For this review, use the dimensioned drawing (mm, ordinates from the lowest corner) and the shaded views. Give positions to 0.01 mm unless a question says otherwise; leave off trailing zeros. Order: outer loops, then holes, each group sorted by start corner. A loop starts at its lowest first (then second) coordinate and runs counter-clockwise, first axis right, second up. Notation, with made-up numbers: (-11.5, 26.5) - (9.5, 26.5) arc R15 cw to (9.5, 55.5) - close; hole circle Ø11 at (33, 66). An arc over 180 degrees is marked (long way). Answer as CSV lines item,"result". Start each with the question number.
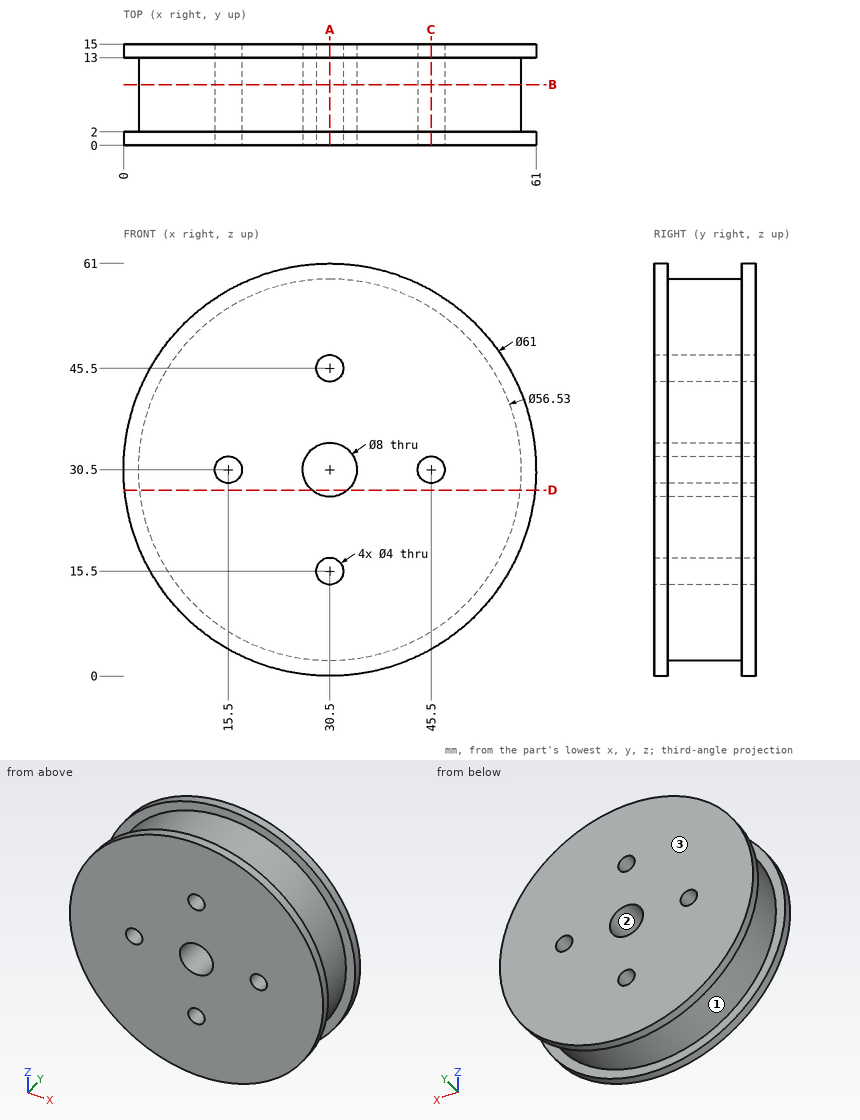
Item 1: For line 1 along X through (y, z) = (12.75, 31); line 2 along X through (y, z) = (3.5, 45.5); line 3 along Y through (x, z) = (22, 3), list the stretches that pass through material, from the lowest coordinate up.
Item 2: Take a section at B-B on y = 9. Write out the cut boundary in (x, z) (3 decimals).
Item 3: Take a section at A-A on x = 30.5. Write out the cut boundary in (y, z) (3 decimals), and give its area (3 significant figures).
Item 4: Take a section at C-C on x = 45.5. Write out the cut boundary in (y, z).
Item 5: Mouldability with a two-part tool opening along Z and no side actions: class the marked faces 1, 2 and 3 as released by +Z, released by -Z, zero draft, split by the parting line, or undercut.
Item 6: Clearance check with flat-ended pins moving along their axes: pin 1 (1.5 mm diameter, centred on y = 9, z = 7, fed in from +X); pin 2 (1.5 mm diameter, centred on x = 48, y = 4.5, fed in from -Z); pin 3 (3 mm diameter, centred on y = 8.5, z = 17.5, fed in from +X). State where each tip first meets the part, or that it passes through.
Item 7: Take a section at D-D on z = 27.5. Write out the cut boundary in (x, y).
Data:
1,line 1,"x = 2.24 to 13.56, 17.44 to 26.53, 34.47 to 43.56, 47.44 to 58.76"
1,line 2,"x = 6.54 to 28.5, 32.5 to 54.46"
1,line 3,"y = 0 to 2, 13 to 15"
2,outline,"circle Ø56.53 at (30.5, 30.5); hole circle Ø4 at (15.5, 30.5); hole circle Ø8 at (30.5, 30.5); hole circle Ø4 at (30.5, 15.5); hole circle Ø4 at (30.5, 45.5); hole circle Ø4 at (45.5, 30.5)"
3,outline,"(0, 0) - (2, 0) - (2, 2.235) - (13, 2.235) - (13, 0) - (15, 0) - (15, 13.5) - (0, 13.5) - close; (0, 17.5) - (15, 17.5) - (15, 26.5) - (0, 26.5) - close; (0, 34.5) - (15, 34.5) - (15, 43.5) - (0, 43.5) - close; (0, 47.5) - (15, 47.5) - (15, 61) - (13, 61) - (13, 58.765) - (2, 58.765) - (2, 61) - (0, 61) - close"
3,area,"626 mm^2"
4,outline,"(0, 3.94) - (2, 3.94) - (2, 6.54) - (13, 6.54) - (13, 3.94) - (15, 3.94) - (15, 28.5) - (0, 28.5) - close; (0, 32.5) - (15, 32.5) - (15, 57.06) - (13, 57.06) - (13, 54.46) - (2, 54.46) - (2, 57.06) - (0, 57.06) - close"
5,face 1,"split by the parting line"
5,face 2,"undercut"
5,face 3,"zero draft"
6,pin 1,"stops at x = 47.27"
6,pin 2,"stops at z = 7.73"
6,pin 3,"stops at x = 56.32"
7,outline,"(0.15, 0) - (27.85, 0) - (27.85, 15) - (0.15, 15) - (0.15, 13) - (2.39, 13) - (2.39, 2) - (0.15, 2) - close; (33.15, 0) - (60.85, 0) - (60.85, 2) - (58.61, 2) - (58.61, 13) - (60.85, 13) - (60.85, 15) - (33.15, 15) - close"
